Part model, mm, in its own coordinate system. A direction names the side the tool comes from. Coordinates: 2 decimals unless noted, no trailing zeros. Write each loop counter-clockwise with the first axis right and the second up, starting at its lowest first coordinate (ties: lowest second). Pieces come first, ordered by that corner, then holes. Notation, with made-up numbers: (25, 49) - (76, 49) arc R13 cw to (76, 68) - close; hole circle Ø7 at (17.5, -2.75). An arc over 180 degrees is marked (long way). Use a Markdown table: item, result.
```python
from build123d import *

# Parameters (mm, degrees)
BOSS_EXTRUDE1_DEPTH        = 6.6294
BOSS_EXTRUDE1_DEPTH_BACK   = 6.6294
F_1_4_0_2500_DOWEL_HOLE1_D = 6.35
F_1_4_0_2500_DOWEL_HOLE2_D = 6.35
FILLET1_R                  = 2.54


with BuildPart() as part:
    # Sketch1 → Boss-Extrude1 (new, two sides: drawn at the far end of the back side and taken through both)
    with BuildSketch(Plane.XY.offset(-BOSS_EXTRUDE1_DEPTH_BACK)):
        Polygon((7.493, 1.016), (7.493, 18.034), (9.525, 18.034), (9.525, -1.016), (-9.525, -1.016), (-9.525, 1.016), align=None)
    extrude(amount=BOSS_EXTRUDE1_DEPTH + BOSS_EXTRUDE1_DEPTH_BACK)

    # 1/4 (0.2500) Dowel Hole1 (through all)
    with Locations(Plane(origin=(0, 1.016, 0), x_dir=(1, 0, 0), z_dir=(0, 1, 0))):
        with Locations((-1.905, 0)):
            Hole(F_1_4_0_2500_DOWEL_HOLE1_D / 2)

    # 1/4 (0.2500) Dowel Hole2 (through all)
    with Locations(Plane.ZY.offset(-7.493)):
        with Locations((0, 10.414)):
            Hole(F_1_4_0_2500_DOWEL_HOLE2_D / 2)

    # Fillet1
    fillet1_edges = [part.edges().sort_by_distance(p)[0] for p in [
        (7.493, 1.016, 0),
        (9.525, -1.016, 0),
    ]]
    fillet(fillet1_edges, radius=FILLET1_R)


solid = part.part
```
Item 1: Drill centre lines: probe 1 along Y at (x, z) = (1.25, -5); probe 2 along Z at (x, y) = (-0.75, 0.75); probe 3 along X at (y, z) = (12.25, 5.5) (3 decimals). Where is each one in solid material? Low to high.
From the geometry:
| item | result |
|---|---|
| probe 1 | -1.02 to 1.02 |
| probe 2 | -6.63 to -2.96, 2.96 to 6.63 |
| probe 3 | 7.493 to 9.525 |
Item 2: Band-saw the part on C-C, the plane z = 4. Give the cut face in (x, y) (3 decimals).
From the geometry:
| item | result |
|---|---|
| outline | (-9.525, -1.016) - (6.985, -1.016) arc R2.54 ccw to (9.525, 1.524) - (9.525, 18.034) - (7.493, 18.034) - (7.493, 3.556) arc R2.54 cw to (4.953, 1.016) - (-9.525, 1.016) - close |
Item 3: Two-plate mould, pull along Z, no slides. Class faces 1 (the face through (8, 4, 6.629)), 2 (the face through (9.525, 8, -3)), 3 (the face through (0.615, -0.014, 1.932)): pulls with the +Z half, pulls with the -Z half, needs draft (parallel to the pull), parting line crosses it, or undercut.
From the geometry:
| item | result |
|---|---|
| face 1 | pulls with the +Z half |
| face 2 | needs draft |
| face 3 | undercut |
Item 4: Drop flat-ended pins along their axis: P1, Ø4, axis at x = -0.5, z = 0, coming from the -Y side; P2, Ø4, axis at y = 13, z = 0.5, coming from the -X side; P3, Ø4, axis at x = -6, z = 3, coming from the +Y side; P4, Ø2, axis at y = 3.5, z = 4.5, coming from the -X side. Give the stop position or say it passes through.
From the geometry:
| item | result |
|---|---|
| P1 | y = -1.02 |
| P2 | x = 7.49 |
| P3 | y = 1.02 |
| P4 | x = 7.26 |
Item 5: Band-saw the part on B-B, the plane y = 7.5. Give the cut face in (x, z) (3 decimals), then the cut area to 3 significant figures.
From the geometry:
| item | result |
|---|---|
| outline | (7.493, -6.629) - (9.525, -6.629) - (9.525, -1.261) - (7.493, -1.261) - close; (7.493, 1.261) - (9.525, 1.261) - (9.525, 6.629) - (7.493, 6.629) - close |
| area | 21.8 mm^2 |
Item 6: Band-saw the part on A-A, the plane z = 0. Give the cut face in (x, y) (3 decimals).
From the geometry:
| item | result |
|---|---|
| outline | (-9.525, -1.016) - (-5.08, -1.016) - (-5.08, 1.016) - (-9.525, 1.016) - close; (1.27, -1.016) - (6.985, -1.016) arc R2.54 ccw to (9.525, 1.524) - (9.525, 7.239) - (7.493, 7.239) - (7.493, 3.556) arc R2.54 cw to (4.953, 1.016) - (1.27, 1.016) - close; (7.493, 13.589) - (9.525, 13.589) - (9.525, 18.034) - (7.493, 18.034) - close |
Item 7: Which spindle directions (+Z, -Z, +X, -X, +Y, -Y) get a long thin tool onto all of the face, cutting with end or side? Do faces 4 (the face through (1, -1.016, -3)), 5 (the face through (7.493, 14, 0)). Say none if no direction does.
From the geometry:
| item | result |
|---|---|
| face 4 | +Z, -Z, +X, -X, -Y |
| face 5 | +Z, -Z, -X, +Y |
Item 8: Band-saw the part on D-D, the plane x = -2. Give the cut face in (y, z), then the cut area to 3 significant figures.
From the geometry:
| item | result |
|---|---|
| outline | (-1.02, -6.63) - (1.02, -6.63) - (1.02, -3.17) - (-1.02, -3.17) - close; (-1.02, 3.17) - (1.02, 3.17) - (1.02, 6.63) - (-1.02, 6.63) - close |
| area | 14.0 mm^2 |
